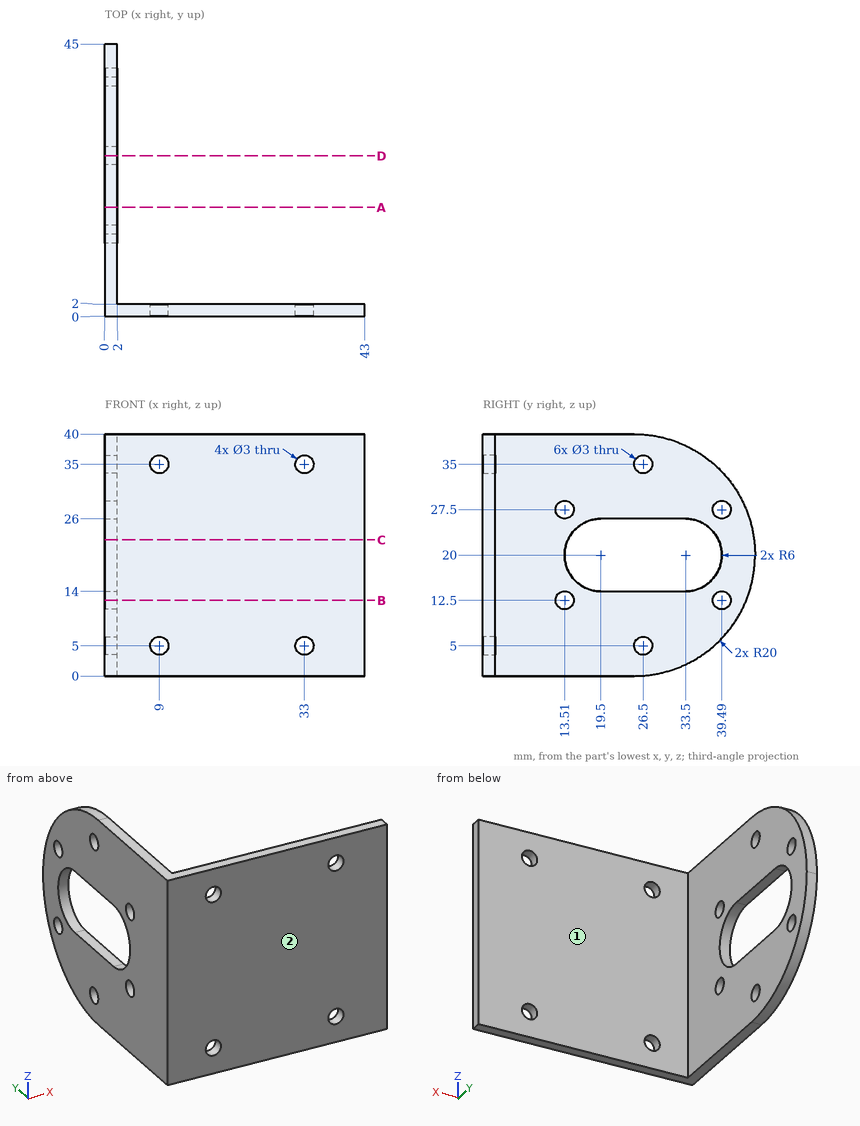
Here's the drawing with two shaded views (mm, measured from the low corner). I have some questions. A direction names the side the tool comes from. Give positions to 0.01 mm unless a question says otherwise; leave off trailing zeros. Loops run counter-clockwise (first coordinate to the right, second up) from the corner with the lowest first, then second, coordinate; pieces in that order, holes last. Notation, with made-up numbers: (31, 81.25) -> (73, 81.25) arc R24 ccw to (73, 105.25) -> close; hole circle Ø2 at (57, -2). An arc over 180 degrees is marked (long way). One line per item, written item: value.
Q1. On a 3-axis mill with a long thin cutter (end or side, diameter ignored), from which of +Z, -Z, +X, -X, +Y, -Y can I reach the whole of each face in a straight line? I mean the marked faces 1 and 2. Say none if no direction works.
Answers follow:
face 1: +Z, -Z, +X, +Y
face 2: +Z, -Z, +X, -X, -Y
Q2. I'm going to push flat-ended pins straight in: pin 1 Ø3.5 at (x, z) = (9, 5) entering from -Y; pin 2 Ø2.5 at (x, z) = (33, 35) entering from +Y; pin 3 Ø8 at (y, z) = (16, 10) entering from +X; pin 4 Ø1 at (x, z) = (33.5, 30) entering from +Y. Where does each tip first touch, or does it pass through?
Answers follow:
pin 1: y = 0
pin 2: through
pin 3: x = 2
pin 4: y = 2
Q3. Suppose I cut it at D-D on y = 26.5. Please give me the cut outline in (x, z).
Answers follow:
outline: (0, 0.06) -> (2, 0.06) -> (2, 3.5) -> (0, 3.5) -> close; (0, 6.5) -> (2, 6.5) -> (2, 14) -> (0, 14) -> close; (0, 26) -> (2, 26) -> (2, 33.5) -> (0, 33.5) -> close; (0, 36.5) -> (2, 36.5) -> (2, 39.94) -> (0, 39.94) -> close
Q4. Suppose I cut it at A-A on y = 18. Please give me the cut outline in (x, z).
Answers follow:
outline: (0, 0) -> (2, 0) -> (2, 14.19) -> (0, 14.19) -> close; (0, 25.81) -> (2, 25.81) -> (2, 40) -> (0, 40) -> close
Q5. Suppose I cut it at C-C on z = 22.5. Please give me the cut outline in (x, y) (1 decimal), then the cut area to 3 significant figures.
Answers follow:
outline: (0, 0) -> (43, 0) -> (43, 2) -> (2, 2) -> (2, 14) -> (0, 14) -> close; (0, 39) -> (2, 39) -> (2, 44.8) -> (0, 44.8) -> close
area: 122 mm^2
Q6. Suppose I cut it at B-B on z = 12.5. Please give me the cut outline in (x, y), then the cut area to 3 significant figures.
Answers follow:
outline: (0, 0) -> (43, 0) -> (43, 2) -> (2, 2) -> (2, 12.01) -> (0, 12.01) -> close; (0, 15.01) -> (2, 15.01) -> (2, 37.99) -> (0, 37.99) -> close; (0, 40.99) -> (2, 40.99) -> (2, 43.54) -> (0, 43.54) -> close
area: 157 mm^2
Q7. If I drill on line 1 along X through (y, z) = (1.35, 35); line 2 along X through (y, z) = (35, 6.5); line 3 along Y through (x, z) = (0.5, 35), over which ranges is the centre line in solid material (lowest first)?
Answers follow:
line 1: 0 to 7.5, 10.5 to 31.5, 34.5 to 43
line 2: 0 to 2
line 3: 0 to 25, 28 to 38.23
